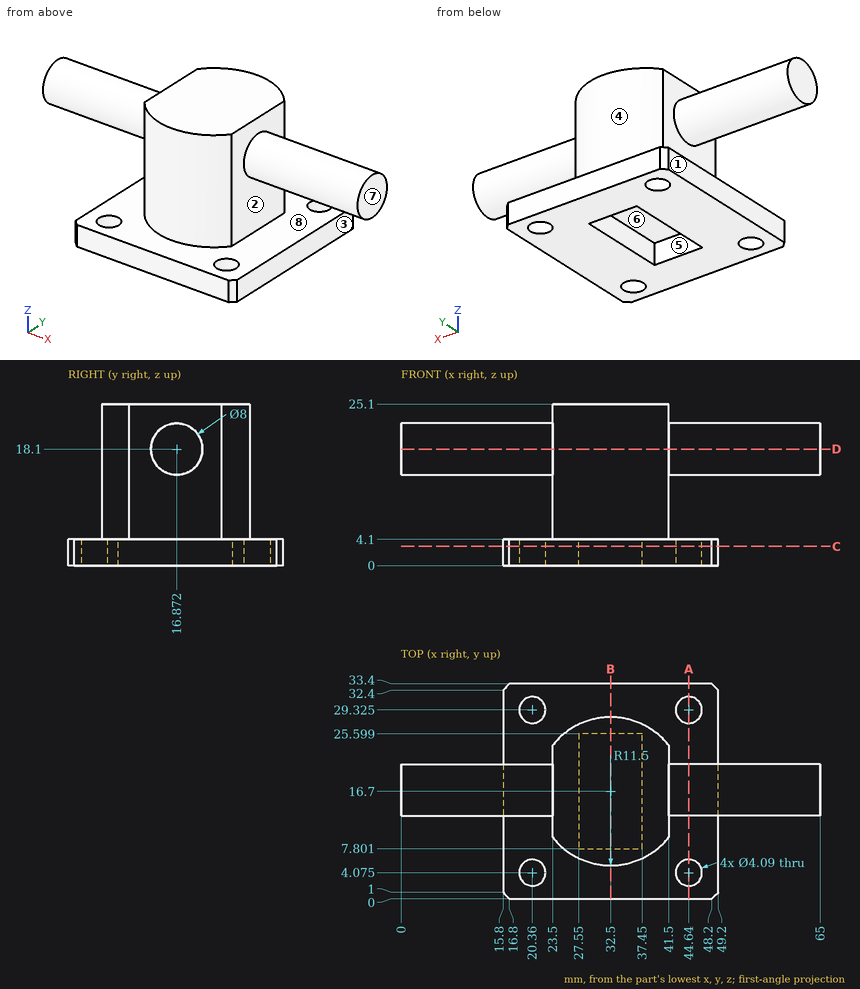
Source: three-view drawing plus pictorial views. Frame: mm from the lowest corner of the part. A direction names the side the tool comes from. Give positions to 0.01 mm unless a question says otherwise; leave off trailing zeros. Order: outer loops, then holes, each group sorted by start corner. A loop starts at its lowest first (then second) coordinate and runs counter-clockwise, first axis right, second up. Notation, with made-up numbers: (-30.75, 56) -> (16.25, 56) arc R17 cw to (16.25, 71) -> close; hole circle Ø6 at (-31.75, 51.5). An arc over 180 degrees is marked (long way). Use a Markdown table: item, result.
Q1. Material intervals for line 1 (Y direction, x = 20.36, z = 1.3); line 2 (Z direction, x = 33, y = 32); line 3 (X direction, y = 16.5, z = 10.25), sorted ascending. Write a range as [from, to].
A:
| item | result |
|---|---|
| line 1 | [0, 2.03], [6.12, 27.28], [31.37, 33.4] |
| line 2 | [0, 4.1] |
| line 3 | [23.5, 41.5] |
Q2. First-contact query: P1, Ø5, axis at y = 29.5, z = 17, coming from the -X side (1 decimal); P2, Ø4, axis at x = 9, z = 12.5, coming from the +Y side (1 decimal); P3, Ø3.5, axis at y = 14, z = 3, coming from the -X side. Flat tips, straight axial feed; report the tip coordinate or a pass-through.
A:
| item | result |
|---|---|
| P1 | x = 27.4 |
| P2 | y = 18.6 |
| P3 | x = 15.8 |
Q3. Section C-C (z = 3). State how many separate pieces and enclosed holes the cut face has, and give its area (3 significant figures).
A:
| item | result |
|---|---|
| separate pieces | 1 |
| enclosed holes | 5 |
| area | 885 mm^2 |
Q4. Section A-A (x = 44.64). Return the cut outline in (y, z), and give its area (3 significant figures).
A:
| item | result |
|---|---|
| outline | (0, 0) -> (2.03, 0) -> (2.03, 4.1) -> (0, 4.1) -> close; (6.12, 0) -> (27.28, 0) -> (27.28, 4.1) -> (6.12, 4.1) -> close; circle Ø8 at (16.87, 18.1); (31.37, 0) -> (33.4, 0) -> (33.4, 4.1) -> (31.37, 4.1) -> close |
| area | 154 mm^2 |
Q5. Access query for the marked faces 1, 2, 3, 4 and 5. Directions: +Z, -Z, +X, -X, +Y, -Y. A direction counts if a zero-diameter tool reaches every point of the face in a straight line with its end or side. Return the directions, or none.
A:
| item | result |
|---|---|
| face 1 | -Z, -X, +Y, -Y |
| face 2 | +X |
| face 3 | -Z, +X, +Y, -Y |
| face 4 | +Z, +Y |
| face 5 | -Z |
Q6. Section D-D (z = 18.1). Return the cut outline in (x, y).
A:
| item | result |
|---|---|
| outline | (0, 12.87) -> (23.5, 12.87) -> (23.5, 9.54) arc R11.5 ccw to (41.5, 9.54) -> (41.5, 12.87) -> (65, 12.87) -> (65, 20.87) -> (41.5, 20.87) -> (41.5, 23.86) arc R11.5 ccw to (23.5, 23.86) -> (23.5, 20.87) -> (0, 20.87) -> close |
Q7. Pull-direction query (X, two-part tool) for the marked faces 6, 7 and 8; classes: +X half, -X half, draft (parallel to the pull), parting line (faces both ways), or undercut.
A:
| item | result |
|---|---|
| face 6 | undercut |
| face 7 | +X half |
| face 8 | draft |
Q8. Section B-B (x = 32.5). Return the cut outline in (y, z).
A:
| item | result |
|---|---|
| outline | (0, 0) -> (7.8, 0) -> (7.8, 4.1) -> (25.6, 4.1) -> (25.6, 0) -> (33.4, 0) -> (33.4, 4.1) -> (28.2, 4.1) -> (28.2, 25.1) -> (5.2, 25.1) -> (5.2, 4.1) -> (0, 4.1) -> close |
